Geometry: final body of the model. Coordinates: model frame, mm. Give positions to 0.01 mm unless a question says otherwise; leave off trailing zeros. Loops run counter-clockwise (first coordinate to the right, second up) from the corner with the lowest first, then second, coordinate; pieces in that order, holes last.
Autodesk Inventor part; units mm, degrees
ref_plane "YZ Plane" through (0, 0, 0) normal (1, 0, 0) x (0, 1, 0)
ref_plane "XZ Plane" through (0, 0, 0) normal (0, 1, 0) x (-1, 0, 0)
ref_plane "XY Plane" through (0, 0, 0) normal (0, 0, 1) x (1, 0, 0)
sketch "Sketch1" plane through (0, 0, 0) normal (0, 1, 0) x (-1, 0, 0)
  line L0 (10, -10) -> (-10, -10) construction
  line L1 (-10, -10) -> (-10, 10) construction
  line L2 (-10, 10) -> (10, 10) construction
  line L3 (10, 10) -> (10, -10) construction
  line L4 (10, -10) -> (-10, 10) construction
  line L5 (-10, -10) -> (10, 10) construction
  line L6 (10, -10) -> (10, -7) construction
  line L7 (11.5, -10) -> (11.5, -7)
  line L8 (8.5, -7) -> (8.5, -10)
  arc A0 (8.5, -10) -> (11.5, -10) centre (10, -10) ccw
  arc A1 (11.5, -7) -> (8.5, -7) centre (10, -7) ccw
  line L9 (-10, -10) -> (-10, -7) construction
  line L10 (-8.5, -10) -> (-8.5, -7)
  line L11 (-11.5, -7) -> (-11.5, -10)
  arc A2 (-11.5, -10) -> (-8.5, -10) centre (-10, -10) ccw
  arc A3 (-8.5, -7) -> (-11.5, -7) centre (-10, -7) ccw
  line L12 (10, 10) -> (10, 13) construction
  line L13 (11.5, 10) -> (11.5, 13)
  line L14 (8.5, 13) -> (8.5, 10)
  arc A4 (8.5, 10) -> (11.5, 10) centre (10, 10) ccw
  arc A5 (11.5, 13) -> (8.5, 13) centre (10, 13) ccw
  line L15 (-10, 10) -> (-10, 13) construction
  line L16 (-8.5, 10) -> (-8.5, 13)
  line L17 (-11.5, 13) -> (-11.5, 10)
  arc A6 (-11.5, 10) -> (-8.5, 10) centre (-10, 10) ccw
  arc A7 (-8.5, 13) -> (-11.5, 13) centre (-10, 13) ccw
  circle A8 centre (14, -20) radius 1.5
  circle A9 centre (-14, -20) radius 1.5
  line L18 (14, -20) -> (-14, -20) construction
  line L19 (18, -24) -> (-18, -24)
  line L20 (-18, -24) -> (-18, -16)
  line L21 (-18, -16) -> (-14, -16)
  line L22 (-14, -16) -> (-14, 17.5)
  line L23 (-14, 17.5) -> (14, 17.5)
  line L24 (14, 17.5) -> (14, -16)
  line L25 (14, -16) -> (18, -16)
  line L26 (18, -16) -> (18, -24)
  point P0 (0, 0)
  point P1 (10, -8.5)
  point P2 (-10, -8.5)
  point P3 (10, 11.5)
  point P4 (-10, 11.5)
  point P5 (0, -20)
  point P6 (0, 0)
  point P7 (0, -24)
  dimension "d0" = 20
  dimension "d1" = 20
  dimension "d2" = 3
  dimension "d3" = 3
  dimension "d4" = 3
  dimension "d5" = 3
  dimension "d6" = 3
  dimension "d7" = 3
  dimension "d8" = 3
  dimension "d9" = 3
  dimension "d10" = 3
  dimension "d11" = 10
  dimension "d12" = 28
  dimension "d13" = 4
  dimension "d15" = 4
  dimension "d16" = 4
  dimension "d17" = 36
  dimension "d18" = 3
extrude "Extrusion1" add sketch "Sketch1" along normal blind 3
fillet "Fillet1" radius 2 8 edges at (14, 1.5, -16) (14, 1.5, 17.5) (-14, 1.5, 17.5) (-14, 1.5, -16) (-18, 1.5, -16) (-18, 1.5, -24) (18, 1.5, -24) (18, 1.5, -16)
properties part number "SecondaryEncoderPCBMount" material "ABS Plastic"
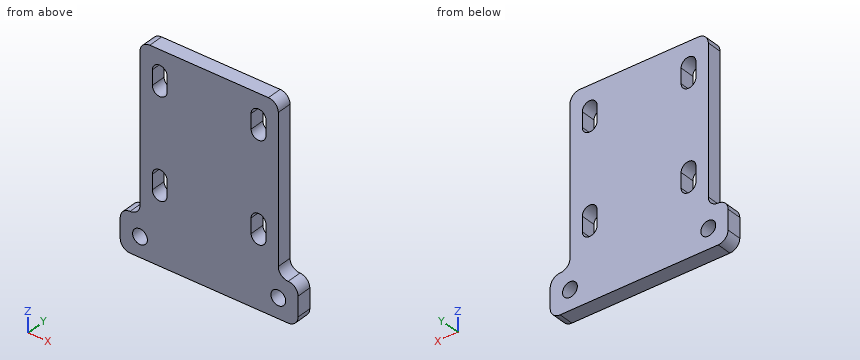
Item 1: Section query A-A on x = -10. Return loops of the section in (y, z), plus the area to 3 significant figures.
Values follow:
outline: (0, -24) - (3, -24) - (3, -11.5) - (0, -11.5) - close; (0, -5.5) - (3, -5.5) - (3, 8.5) - (0, 8.5) - close; (0, 14.5) - (3, 14.5) - (3, 17.5) - (0, 17.5) - close
area: 88.5 mm2
Item 2: Section query C-C on z = -13. Return loops of the section in (x, y).
Values follow:
outline: (-14, 0) - (14, 0) - (14, 3) - (-14, 3) - close
Item 3: Ray query, probe 1 along X at (y, z) = (2.85, -2.5); probe 2 along X at (y, z) = (2.8, 13.5). Return the intervals inside material, ascending.
Values follow:
probe 1: x = -14 to 14
probe 2: x = -14 to -11.41, -8.59 to 8.59, 11.41 to 14
Item 4: Section query B-B on z = 12. Return loops of the section in (x, y).
Values follow:
outline: (-14, 0) - (-11.5, 0) - (-11.5, 3) - (-14, 3) - close; (-8.5, 0) - (8.5, 0) - (8.5, 3) - (-8.5, 3) - close; (11.5, 0) - (14, 0) - (14, 3) - (11.5, 3) - close
Item 5: Pin query (flat end, axial travel): pin 1 (1.5 mm diameter, centred on y = 2, z = 11.5, fed in from +X); pin 2 (1.5 mm diameter, centred on y = 1, z = -9, fed in from -X). Return the tip coordinate at first contact, or that it passes through.
Values follow:
pin 1: stops at x = 14
pin 2: stops at x = -14
